Build history of the part. All positions in model axes, mm. Face numbers are marked on the shaded views. A direction names the side the tool comes from. Round coordinates to 2 decimals unless told otherwise and drop trailing zeros. Write each loop counter-clockwise with the first axis right and the second up, starting at its lowest first coordinate (ties: lowest second). Pieces come first, ordered by that corner, then holes. Notation, with made-up numbers: (-15.5, 64.5) -> (4.5, 64.5) arc R27 ccw to (4.5, 93.5) -> close; hole circle Ø4 at (18, 64.5). An arc over 180 degrees is marked (long way). Answer in a Markdown table with one row per item. Add a question column.
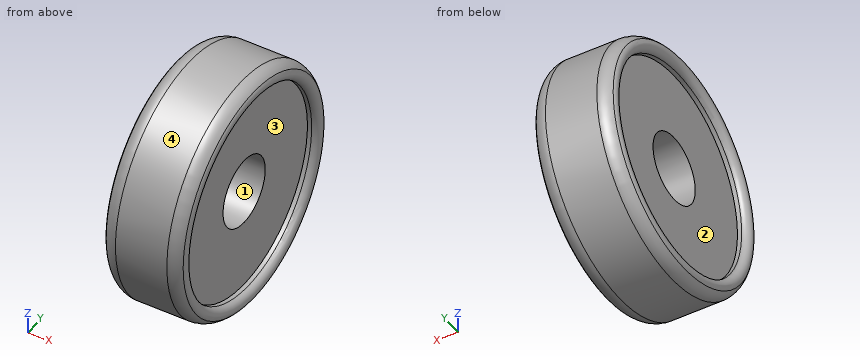
from build123d import *

# Parameters (mm, degrees)
SKETCH1_R           = 350
SKETCH1_R_2         = 100
BOSS_EXTRUDE1_DEPTH = 125
FILLET1_R           = 50
FILLET2_R           = 50
SKETCH2_R           = 300
CUT_EXTRUDE1_DEPTH  = 40
CUT_EXTRUDE2_START  = -40
SKETCH4_R           = 300
CUT_EXTRUDE2_DEPTH  = 40
FILLET3_R           = 20
FILLET4_R           = 20


with BuildPart() as part:
    # Sketch1 → Boss-Extrude1 (new, symmetric)
    with BuildSketch(Plane(origin=(0, 0, 0), x_dir=(0, 0, -1), z_dir=(1, 0, 0))):
        Circle(SKETCH1_R)
        Circle(SKETCH1_R_2, mode=Mode.SUBTRACT)
    extrude(amount=BOSS_EXTRUDE1_DEPTH, both=True)

    # Fillet1
    fillet1_edges = [part.edges().sort_by_distance(p)[0] for p in [
        (-125, 0, 350),
    ]]
    fillet(fillet1_edges, radius=FILLET1_R)

    # Fillet2
    fillet2_edges = [part.edges().sort_by_distance(p)[0] for p in [
        (125, 0, 350),
    ]]
    fillet(fillet2_edges, radius=FILLET2_R)

    # Sketch2 → Cut-Extrude1 (cut)
    with BuildSketch(Plane.ZY.offset(125)):
        Circle(SKETCH2_R)
    extrude(amount=-CUT_EXTRUDE1_DEPTH, mode=Mode.SUBTRACT)

    # Sketch4 → Cut-Extrude2 (cut)
    with BuildSketch(Plane(origin=(125, 0, 0), x_dir=(0, 0, -1), z_dir=(1, 0, 0)).offset(CUT_EXTRUDE2_START)):
        with Locations(Location((0, 0, 0), (0, 0, 180))):
            Circle(SKETCH4_R)
    extrude(amount=CUT_EXTRUDE2_DEPTH, mode=Mode.SUBTRACT)

    # Fillet3
    # the kernel refuses this fillet: 20 mm, written as the material it takes off along each edge
    with BuildSketch(Plane(origin=(125, 0, 0), x_dir=(0, 0, -1), z_dir=(0, -1, 0))) as fillet3_piece_1:
        with BuildLine():
            CenterArc((320, -27.639320225), FILLET3_R, 48.189685104, 131.810314896)
            Line((300, -27.639320225), (300, 0))
            ThreePointArc((300, 0), (317.841104489, -3.291382052), (333.333333333, -12.732200375))
        make_face()
    fillet3_piece_1_solid = revolve(axis=Axis((125, 0, 0), (1, 0, 0)), revolution_arc=180, mode=Mode.PRIVATE)
    with BuildSketch(Plane(origin=(125, 0, 0), x_dir=(0, 0, 1), z_dir=(0, 1, 0))) as fillet3_piece_2:
        with BuildLine():
            CenterArc((320, -27.639320225), FILLET3_R, 48.189685104, 131.810314896)
            Line((300, -27.639320225), (300, 0))
            ThreePointArc((300, 0), (317.841104489, -3.291382052), (333.333333333, -12.732200375))
        make_face()
    fillet3_piece_2_solid = revolve(axis=Axis((125, 0, 0), (1, 0, 0)), revolution_arc=180, mode=Mode.PRIVATE)
    add([fillet3_piece_1_solid, fillet3_piece_2_solid], mode=Mode.SUBTRACT)

    # Fillet4
    # the kernel refuses this fillet: 20 mm, written as the material it takes off along each edge
    with BuildSketch(Plane(origin=(-125, 0, 0), x_dir=(0, 0, -1), z_dir=(0, -1, 0))) as fillet4_piece_1:
        with BuildLine():
            CenterArc((320, 27.639320225), FILLET4_R, 180, 131.810314896)
            Line((300, 27.639320225), (300, 0))
            ThreePointArc((300, 0), (317.841104489, 3.291382052), (333.333333333, 12.732200375))
        make_face()
    fillet4_piece_1_solid = revolve(axis=Axis((-125, 0, 0), (1, 0, 0)), revolution_arc=180, mode=Mode.PRIVATE)
    with BuildSketch(Plane(origin=(-125, 0, 0), x_dir=(0, 0, 1), z_dir=(0, 1, 0))) as fillet4_piece_2:
        with BuildLine():
            CenterArc((320, 27.639320225), FILLET4_R, 180, 131.810314896)
            Line((300, 27.639320225), (300, 0))
            ThreePointArc((300, 0), (317.841104489, 3.291382052), (333.333333333, 12.732200375))
        make_face()
    fillet4_piece_2_solid = revolve(axis=Axis((-125, 0, 0), (1, 0, 0)), revolution_arc=180, mode=Mode.PRIVATE)
    add([fillet4_piece_1_solid, fillet4_piece_2_solid], mode=Mode.SUBTRACT)


solid = part.part
(1) Saw through at C-C (x = -18). List the corners of the cut face in (y, z), plus the area to 3 significant figures.
(2) Which spindle directions (+Z, -Z, +X, -X, +Y, -Y) get a long thin tool onto all of the face, cutting with end or side? Do the marked faces 1 and 2. Say none if no direction does.
(3) Mould opens along Y. For the marked faces 3 and 4 say: pulls with the +Y half, pulls with the -Y half, needs draft (parallel to the pull), parting line crosses it, or undercut.
(4) Drop flat-ended pins along their axis: P1, Ø4, axis at x = 15.5, z = 243, coming from the -Y side; P2, Ø4, axis at y = -220, z = -226.5, coming from the +X side; P3, Ø10, axis at y = -25, z = 261.5, coming from the +X side. Give the stop position or say it passes through.
(5) Saw through at A-A (z = 0). List the corners of the cut face in (x, y).
(6) Probe line 1 along X through (y, z) = (-139, -75); line 2 along Y through (x, z) = (-89, 0); line 3 along Y through (x, z) = (-76, 36). List the from-to ranges inside material, lowest first.
Answer sheet:
| question | item | result |
|---|---|---|
| 1 | outline | circle Ø700 at (0, 0); hole circle Ø200 at (0, 0) |
| 1 | area | 353,000 mm² |
| 2 | face 1 | +X, -X |
| 2 | face 2 | -X |
| 3 | face 3 | undercut |
| 3 | face 4 | parting line crosses it |
| 4 | P1 | stops at y = -253.81 |
| 4 | P2 | stops at x = 117.23 |
| 4 | P3 | stops at x = 85 |
| 5 | outline | (-112.27, -333.33) arc R50 ccw to (-75, -350) -> (75, -350) arc R50 ccw to (112.27, -333.33) arc R20 ccw to (97.36, -300) -> (85, -300) -> (85, -100) -> (-85, -100) -> (-85, -300) -> (-97.36, -300) arc R20 ccw to start; (-112.27, 333.33) arc R20 ccw to (-97.36, 300) -> (-85, 300) -> (-85, 100) -> (85, 100) -> (85, 300) -> (97.36, 300) arc R20 ccw to (112.27, 333.33) arc R50 ccw to (75, 350) -> (-75, 350) arc R50 ccw to start |
| 6 | line 1 | x = -85 to 85 |
| 6 | line 2 | y = -348 to -300, 300 to 348 |
| 6 | line 3 | y = -348.13 to -93.3, 93.3 to 348.13 |
